from build123d import *

# Parameters (mm, degrees)
F0_W           = 129.58
F0_H           = 66
F1_DEPTH       = 10
F3_D           = 3
F3_DEPTH       = 11
F3_CBORE_D     = 5.5
F3_CBORE_DEPTH = 2
F3_TIP         = 0.9012909285
F4_T           = 2
F5_R           = 1


# Not quite as in the source:
# - a shell that OpenCascade refuses in one call is made with other operations: the cavity is built on its own and cut out


with BuildPart() as f1:
    # F0 (on Front) → F1 (new body)
    with BuildSketch(Plane.XZ):
        with Locations((64.79, 33)):
            Rectangle(F0_W, F0_H)
    extrude(amount=F1_DEPTH)

    # F3
    with Locations(Plane(origin=(0, 0, 0), x_dir=(1, 0, 0), z_dir=(0, 1, 0))):
        with Locations((4, -62), (4, -4), (125.58, -4), (125.58, -62)):
            CounterBoreHole(F3_D / 2, F3_CBORE_D / 2, F3_CBORE_DEPTH, depth=F3_DEPTH)
            with Locations((0, 0, -(F3_DEPTH + F3_TIP / 2))):  # 118° drill point
                Cone(0, F3_D / 2, F3_TIP, mode=Mode.SUBTRACT)

    # F4: shell of thickness 2, made by hand


with BuildPart() as f4_core1:
    # F4_t2: copy of F1
    add(f1.part)

    # the walls: a layer under each face that stays
    f4_faces = [f4_core1.faces().sort_by_distance(p)[0] for p in [
        (0, -5, 33),
        (64.79, -5, 66),
        (64.79, -5, 0),
        (64.79, 0, 33),
        (129.58, -5, 33),
        (1.25, -1, 4),
        (122.83, -1, 4),
        (1.25, -1, 62),
        (122.83, -1, 62),
        (2.5, -6, 4),
        (124.08, -6, 4),
        (2.5, -6, 62),
        (124.08, -6, 62),
        (2.1666666667, -2, 5.8333333333),
        (123.7466666667, -2, 5.8333333333),
        (2.1666666667, -2, 63.8333333333),
        (123.7466666667, -2, 63.8333333333),
    ]]
    thicken(f4_faces, amount=-F4_T, mode=Mode.SUBTRACT)

    # F4_s3 → F4_t4 (revolve, cut)
    with BuildSketch(Plane.XY.offset(4)):
        Polygon((6.73, -1.98), (8.75, -2), (8.75, -4), (6.75, -4), align=None)
    revolve(axis=Axis((4, -2, 4), (0, 1, 0)), mode=Mode.SUBTRACT)

    # F4_s5 → F4_t6 (revolve, cut)
    with BuildSketch(Plane.XY.offset(4)):
        Polygon((128.31, -1.98), (130.33, -2), (130.33, -4), (128.33, -4), align=None)
    revolve(axis=Axis((125.58, -2, 4), (0, 1, 0)), mode=Mode.SUBTRACT)

    # F4_s7 → F4_t8 (revolve, cut)
    with BuildSketch(Plane.XY.offset(62)):
        Polygon((6.73, -1.98), (8.75, -2), (8.75, -4), (6.75, -4), align=None)
    revolve(axis=Axis((4, -2, 62), (0, 1, 0)), mode=Mode.SUBTRACT)

    # F4_s9 → F4_t10 (revolve, cut)
    with BuildSketch(Plane.XY.offset(62)):
        Polygon((128.31, -1.98), (130.33, -2), (130.33, -4), (128.33, -4), align=None)
    revolve(axis=Axis((125.58, -2, 62), (0, 1, 0)), mode=Mode.SUBTRACT)


with BuildPart() as f1_1:
    add(f1.part)

    # what is left inside the walls is the cavity
    f4_cavity = [f4_core1.part.solids().sort_by_distance(p)[0] for p in [
        (64.79, -9.98, 22.666667),
    ]]
    add(f4_cavity, mode=Mode.SUBTRACT)

    # F5
    f5_edges = [f1_1.edges().sort_by_distance(p)[0] for p in [
        (129.58, 0, 33),
        (64.79, 0, 66),
        (0, 0, 33),
        (64.79, 0, 0),
        (129.58, -5, 66),
        (129.58, -5, 0),
        (0, -5, 0),
        (0, -5, 66),
    ]]
    fillet(f5_edges, radius=F5_R)


solid = f1_1.part
Build history of the part. All positions in model axes, mm. A direction names the side the tool comes from. Coordinates: 2 decimals unless noted, no trailing zeros. Order: outer loops, then holes, each group sorted by start corner. A loop starts at its lowest first (then second) coordinate and runs counter-clockwise, first axis right, second up. Notation, with made-up numbers: (75, 9) - (108, 9) arc R34 ccw to (108, 47) - close; hole circle Ø7 at (-35.75, -20). An arc over 180 degrees is marked (long way). Write item = value, one per line. Start each with the question number.
1) Two-plate mould, pull along X, no slides. Class faces 1 (the face through (129.58, -5, 33)), 2 (the face through (2, -6, 33)), 3 (the face through (0, -5, 33)), 4 (the face through (64, 0, 33)): pulls with the +X half, pulls with the -X half, needs draft (parallel to the pull), parting line crosses it, or undercut.
2) Saw through at A-A on z = 62. Count the separate pieces of the cut face and the enclosed holes in it, then the cut area to 3 significant figures.
3) 3-axis set-ups, long thin cutter, end or side, ignore diameter. For faces 5 (the face through (3.642, -0.986, 59.273)), 6 (the face through (123, -4, 7)), 7 (the face through (60, -10, 65)): which of +Z, -Z, +X, -X, +Y, -Y reach the whole face in a straight line?
4) Flat gauge pins, fed straight in: pin 1 Ø2 at (x, z) = (125, 61) entering from -Y; pin 2 Ø4 at (x, z) = (29, 37.5) entering from -Y; pin 3 Ø5 at (x, z) = (125.58, 4) entering from +Y. Where does each tip first touch, or does it go through?
5) Saw through at D-D on z = 36. Write the cut outline in (x, y).
6) Wall check: line 1 along Z through (x, y) = (125.58, -1.4); line 2 along Z through (x, y) = (4, -5.5); line 3 along X through (y, z) = (-7.75, 4). Give the ranges that are in metal, low to high. Write a range as from..to.
7) Saw through at C-C on y = -5.75. Write the cut outline in (x, z), then the cut area to 3 significant figures.
From the geometry:
q1.face_1 = pulls with the +X half
q1.face_2 = undercut
q1.face_3 = pulls with the -X half
q1.face_4 = needs draft
q2.separate_pieces = 3
q2.enclosed_holes = 0
q2.area = 314 mm^2
q3.face_5 = +Y
q3.face_6 = -Y
q3.face_7 = +Z, -Z, +X, -X, -Y
q4.pin_1 = -10
q4.pin_2 = -2
q4.pin_3 = -2
q5.outline = (0, -10) - (2, -10) - (2, -2) - (127.58, -2) - (127.58, -10) - (129.58, -10) - (129.58, -1) arc R1 ccw to (128.58, 0) - (1, 0) arc R1 ccw to (0, -1) - close
q6.line_1 = 0..1.25, 6.75..59.25, 64.75..66
q6.line_2 = 0..2.5, 5.5..7.5, 58.5..60.5, 63.5..66
q6.line_3 = 0..2.5, 5.5..7.5, 122.08..124.08, 127.08..129.58
q7.outline = (0, 1) arc R1 ccw to (1, 0) - (128.58, 0) arc R1 ccw to (129.58, 1) - (129.58, 65) arc R1 ccw to (128.58, 66) - (1, 66) arc R1 ccw to (0, 65) - close; hole (2, 6.87) arc R3.5 cw to (6.87, 2) - (122.71, 2) arc R3.5 cw to (127.58, 6.87) - (127.58, 59.13) arc R3.5 cw to (122.71, 64) - (6.87, 64) arc R3.5 cw to (2, 59.13) - close; hole circle Ø3 at (4, 4); hole circle Ø3 at (4, 62); hole circle Ø3 at (125.58, 4); hole circle Ø3 at (125.58, 62)
q7.area = 844 mm^2
